Verification items for the finished model (mm, model axes). A direction names the side the tool comes from. Give positions to 0.01 mm unless a question says otherwise; leave off trailing zeros. Loops run counter-clockwise (first coordinate to the right, second up) from the corner with the lowest first, then second, coordinate; pieces in that order, holes last. Notation, with made-up numbers: M 20.5,58.5 L 35.5,58.5 A25 cw 35.5,97.5 Z; hole C 21,8.5 d5. An arc over 180 degrees is marked long. Use a Markdown table: item, result.
from build123d import *

# Parameters (mm, degrees)
F0_W      = 60
F0_H      = 40
F1_DEPTH  = 4
F3_DEPTH  = 60
F4_W      = 2.2
F4_H      = 2.2
F4_W_2    = 2.5
F4_H_2    = 2.3
F5_DEPTH  = 60
F4_H_3    = 0.7
F6_DEPTH  = 60
F7_W      = 25
F7_H      = 2.2
F8_DEPTH  = 2.2
F9_W      = 26
F9_H      = 2.5
F10_DEPTH = 1.7
F11_SIZE  = 0.5


with BuildPart() as f1:
    # F0 (on Top) → F1 (new body)
    with BuildSketch(Plane.XY):
        Rectangle(F0_W, F0_H)
    extrude(amount=F1_DEPTH)

    # F2 (on face) → F3 (join, through all)
    with BuildSketch(Plane.YZ.offset(30)):
        Polygon((12, 53.300871376), (3.6678885292, 4), (15, 4), (15, 53.300871376), align=None)
        Polygon((-20, 8), (-20, 4), (3.6678885292, 4), align=None)
    extrude(amount=-F3_DEPTH)

    # F4 (on face) → F5 (cut, through all)
    with BuildSketch(Plane.YZ.offset(30)):
        with Locations((-18.9, 1.1)):
            Rectangle(F4_W, F4_H)
        Polygon((-17.8, 2.2), (-17.8, 0), (-15, 0), (-15, 5), (-17.8, 5), align=None)
        with Locations((16.25, 2.85)):
            Rectangle(F4_W_2, F4_H_2)
    extrude(amount=-F5_DEPTH, mode=Mode.SUBTRACT)

    # F4 (on face) → F6 (join, through all)
    with BuildSketch(Plane.YZ.offset(30)):
        with Locations((18.75, 4.35)):
            Rectangle(F4_W_2, F4_H_3)
    extrude(amount=-F6_DEPTH)

    # F7 (on face) → F8 (join, through all)
    with BuildSketch(Plane(origin=(0, 0, 2.2), x_dir=(1, 0, 0), z_dir=(0, 0, -1))):
        with Locations((0, 18.9)):
            Rectangle(F7_W, F7_H)
    extrude(amount=F8_DEPTH)

    # F9 (on face) → F10 (cut, through all)
    with BuildSketch(Plane.XY.offset(1.7)):
        with Locations((0, 16.25)):
            Rectangle(F9_W, F9_H)
    extrude(amount=-F10_DEPTH, mode=Mode.SUBTRACT)

    # F11
    f11_edges = [f1.edges().sort_by_distance(p)[0] for p in [
        (0, 20, 4.7),
        (0, 17.5, 4.7),
        (-13, 16.25, 1.7),
        (13, 16.25, 1.7),
    ]]
    chamfer(f11_edges, length=F11_SIZE)


solid = f1.part
(1) Cross-section at B-B on x = -21.5. Record the cut outline in (y, z), then the cut area to 3 significant figures.
Results below:
| item | result |
|---|---|
| outline | M -20,2.2 L -17.8,2.2 L -17.8,5 L -15,5 L -15,0 L 20,0 L 20,4.2 L 19.5,4.7 L 18,4.7 L 17.5,4.2 L 17.5,1.7 L 15,1.7 L 15,53.3 L 12,53.3 L 3.67,4 L -20,8 Z |
| area | 538 mm^2 |
(2) Gauge pin test, flat ends, axial feed: P1, Ø0.7, axis at x = 19, y = -18.5, coming from the -Z side; P2, Ø1.4, axis at x = -8, y = -16.5, coming from the -Z side; P3, Ø1.2, axis at x = 22, y = 16.5, coming from the +Z side. Record the tip position at first contact, or that the pin passes through.
Results below:
| item | result |
|---|---|
| P1 | z = 2.2 |
| P2 | z = 5 |
| P3 | z = 1.7 |
(3) Cross-section at D-D on y = -16. Record the cut outline in (x, z), then the cut area to 3 significant figures.
Results below:
| item | result |
|---|---|
| outline | M -30,5 L 30,5 L 30,7.32 L -30,7.32 Z |
| area | 139 mm^2 |
(4) Cross-section at C-C on z = 22. Record the cut outline in (x, y).
Results below:
| item | result |
|---|---|
| outline | M -30,6.71 L 30,6.71 L 30,15 L -30,15 Z |
(5) Set-up check for faces 4 (the flat face through (0, 19, 4.7)), 5 (the flat face through (-21, -19, 2.2)), 6 (the flat face through (0.42, -8, 5.97)), 7 (the flat face through (0, -16, 5)), 8 (the flat face through (21, -19, 2.2)): record each of +Z, -Z, +X, -X, +Y, -Y from which the full face is reachable in a straight line by a thin tool's end or side.
Results below:
| item | result |
|---|---|
| face 4 | +Z, +X, -X, +Y |
| face 5 | -Z, -X, -Y |
| face 6 | +Z, +X, -X |
| face 7 | -Z, +X, -X |
| face 8 | -Z, +X, -Y |
(6) Draft check along Y on faces 1 (the flat face through (22, 16, 1.7)), 2 (the flat face through (0, 20, 2)), 3 (the flat face through (-30, 7, 17)). Enter one of: +Y half, -Y half, draft (parallel to the pull), parting line (faces both ways), or undercut.
Results below:
| item | result |
|---|---|
| face 1 | undercut |
| face 2 | +Y half |
| face 3 | draft |
(7) Material ranges on line 1 (Y direction, x = -12.5, z = 34.5); line 2 (Y direction, x = 6.5, z = 11.5); line 3 (Z direction, x = -3, y = -10.5), recorded low to high.
Results below:
| item | result |
|---|---|
| line 1 | 8.82 to 15 |
| line 2 | 4.94 to 15 |
| line 3 | 0 to 6.39 |
(8) Cross-section at A-A on x = 11.5. Record the cut outline in (y, z), then the cut area to 3 significant figures.
Results below:
| item | result |
|---|---|
| outline | M -20,0 L -17.8,0 L -17.8,5 L -15,5 L -15,0 L 15,0 L 15,53.3 L 12,53.3 L 3.67,4 L -20,8 Z; M 17.5,0 L 20,0 L 20,4.2 L 19.5,4.7 L 18,4.7 L 17.5,4.2 Z |
| area | 538 mm^2 |
